Autodesk Inventor part; units mm, degrees
ref_plane "YZ Plane" through (0, 0, 0) normal (1, 0, 0) x (0, 1, 0)
ref_plane "XZ Plane" through (0, 0, 0) normal (0, 1, 0) x (-1, 0, 0)
ref_plane "XY Plane" through (0, 0, 0) normal (0, 0, 1) x (1, 0, 0)
sketch "Skizze1" plane through (0, 0, 0) normal (0, 1, 0) x (-1, 0, 0)
  line L0 (0, 0) -> (-110, 0)
  line L1 (-110, 0) -> (-110, 98)
  line L2 (-110, 98) -> (0, 98)
  line L3 (0, 98) -> (0, 0)
  dimension "d0" = 110
  dimension "d1" = 98
extrude "Extrusion1" add sketch "Skizze1" along normal blind 5
sketch "Skizze2" plane through (0, 0, 0) normal (0, -1, 0) x (1, 0, 0)
  line L0 (107, 93) -> (105, 93)
  line L1 (105, 93) -> (105, 36)
  line L2 (105, 36) -> (107, 36)
  line L3 (107, 36) -> (107, 93)
  line L4 (3, 93) -> (5, 93)
  line L5 (5, 93) -> (5, 36)
  line L6 (5, 36) -> (3, 36)
  line L7 (3, 36) -> (3, 93)
  line L8 (5, 36) -> (9, 36)
  line L9 (9, 36) -> (9, 38)
  line L10 (9, 38) -> (5, 38)
  line L11 (5, 38) -> (5, 36)
  line L12 (5, 93) -> (9, 93)
  line L13 (9, 93) -> (9, 91)
  line L14 (9, 91) -> (5, 91)
  line L15 (5, 91) -> (5, 93)
  line L16 (105, 93) -> (101, 93)
  line L17 (101, 93) -> (101, 91)
  line L18 (101, 91) -> (105, 91)
  line L19 (105, 91) -> (105, 93)
  line L20 (105, 36) -> (101, 36)
  line L21 (101, 36) -> (101, 38)
  line L22 (101, 38) -> (105, 38)
  line L23 (105, 38) -> (105, 36)
extrude "Extrusion2" add sketch "Skizze2" along normal blind 8 contours L3 L2 L1 L0
extrude "Extrusion3" add sketch "Skizze2" along normal blind 8 contours L20 L21 L22 L1
extrude "Extrusion4" add sketch "Skizze2" along normal blind 8 contours L1 L18 L17 L16
extrude "Extrusion5" add sketch "Skizze2" along normal blind 8 contours L5 L10 L9 L8
extrude "Extrusion6" add sketch "Skizze2" along normal blind 8 contours L4 L5 L6 L7
extrude "Extrusion7" add sketch "Skizze2" along normal blind 8 contours L12 L13 L14 L5
sketch "Skizze3" plane through (0, -8, 0) normal (0, -1, 0) x (1, 0, 0)
  line L0 (5, 38) -> (5, 91)
  line L1 (3, 93) -> (3, 36)
  line L2 (3, 80) -> (5, 80)
  line L3 (5, 80) -> (5, 50)
  line L4 (5, 50) -> (3, 50)
  line L5 (3, 50) -> (3, 80)
  point P0 (0, 0)
extrude "Extrusion8" cut sketch "Skizze3" against normal blind 8
sketch "Skizze4" plane through (0, 5, 0) normal (0, 1, 0) x (1, 0, 0)
  line L0 (12.0049, -91) -> (87.0387, -91)
  line L1 (87.0387, -91) -> (87.0387, -37.9492)
  line L2 (87.0387, -37.9492) -> (12.0049, -37.9492)
  line L3 (12.0049, -37.9492) -> (12.0049, -91)
extrude "Extrusion9" cut sketch "Skizze4" against normal blind 8
sketch "Skizze5" plane through (0, 0, 0) normal (0, -1, 0) x (1, 0, 0)
  line L0 (3, 3) -> (107, 3)
  line L1 (107, 3) -> (107, 30)
  line L2 (107, 30) -> (3, 30)
  line L3 (3, 30) -> (3, 3)
extrude "Extrusion10" add sketch "Skizze5" along normal blind 10
sketch "Skizze6" plane through (0, -10, 0) normal (0, -1, 0) x (1, 0, 0)
  line L0 (5, 5) -> (105, 5)
  line L1 (105, 5) -> (105, 28)
  line L2 (105, 28) -> (5, 28)
  line L3 (5, 28) -> (5, 5)
  point P0 (0, 0)
extrude "Extrusion11" cut sketch "Skizze6" against normal blind 10
sketch "Skizze7" plane through (0, -10, 0) normal (0, -1, 0) x (1, 0, 0)
  line L0 (107, 30) -> (3, 30)
  line L1 (5, 28) -> (105, 28)
  line L2 (14, 30) -> (98, 30)
  line L3 (98, 30) -> (98, 28)
  line L4 (98, 28) -> (14, 28)
  line L5 (14, 28) -> (14, 30)
  point P0 (0, 0)
extrude "Extrusion12" cut sketch "Skizze7" against normal blind 10
sketch "Skizze8" plane through (0, -10, 0) normal (0, -1, 0) x (1, 0, 0)
  line L0 (105, 5) -> (5, 5)
  line L1 (107, 3) -> (3, 3)
  line L2 (16, 5) -> (96, 5)
  line L3 (96, 5) -> (96, 3)
  line L4 (96, 3) -> (16, 3)
  line L5 (16, 3) -> (16, 5)
  point P0 (0, 0)
extrude "Extrusion13" cut sketch "Skizze8" against normal blind 10
sketch "Skizze14" plane through (0, 0, 0) normal (0, -1, 0) x (1, 0, 0)
  line L0 (87.0387, 37.9492) -> (98, 37.9492)
  line L1 (98, 37.9492) -> (98, 91)
  line L2 (98, 91) -> (87.0387, 91)
  line L3 (87.0387, 91) -> (87.0387, 37.9492)
extrude "Extrusion20" cut sketch "Skizze14" against normal blind 2
sketch "Skizze15" plane through (0, 0, 0) normal (0, -1, 0) x (1, 0, 0)
  line L0 (104, 6) -> (6, 6)
  line L1 (6, 6) -> (6, 27)
  line L2 (6, 27) -> (104, 27)
  line L3 (104, 27) -> (104, 6)
extrude "Extrusion21" cut sketch "Skizze15" against normal blind 3
sketch "Skizze16" plane through (0, -10, 0) normal (0, -1, 0) x (1, 0, 0)
  line L0 (104, 28) -> (6, 28)
  line L1 (6, 28) -> (6, 30)
  line L2 (6, 30) -> (104, 30)
  line L3 (104, 30) -> (104, 28)
  point P0 (0, 0)
extrude "Extrusion22" cut sketch "Skizze16" against normal blind 10
sketch "Skizze17" plane through (0, 0, 0) normal (0, -1, 0) x (1, 0, 0)
  line L0 (9, 36) -> (3, 36)
  line L1 (104, 27) -> (6, 27)
  line L2 (6, 27) -> (6, 36)
  line L3 (6, 36) -> (104, 36)
  line L4 (104, 36) -> (104, 27)
extrude "Extrusion23" cut sketch "Skizze17" against normal blind 3
sketch "Skizze18" plane through (0, 0, 0) normal (0, -1, 0) x (1, 0, 0)
  line L0 (12.0049, 91) -> (12.0049, 37.9492)
  line L1 (12.0049, 39) -> (6, 39)
  line L2 (6, 39) -> (6, 90)
  line L3 (6, 90) -> (12.0049, 90)
  line L4 (12.0049, 90) -> (12.0049, 39)
extrude "Extrusion24" cut sketch "Skizze18" against normal blind 3
properties part number "ARDUINO_DUE_CASE_TOP_NEU"
Build history of the part. All positions in model axes, mm. A direction names the side the tool comes from. Round coordinates to 2 decimals unless told otherwise and drop trailing zeros. Loops run counter-clockwise (first coordinate to the right, second up) from the corner with the lowest first, then second, coordinate; pieces in that order, holes last. Notation, with made-up numbers: M 32.5,-22.5 L 51.5,-22.5 A15 cw 51.5,5.5 Z; hole C 46.25,9.5 d4. An arc over 180 degrees is marked long. Answer as CSV lines item,"result".
1. Wall check: probe 1 along Z at (x, y) = (68, 0.5); probe 2 along X at (y, z) = (-5, 82.5); probe 3 along X at (y, z) = (1.5, 75). Give the ranges that are in metal, low to high. Write a range as [from, to].
Resolved:
probe 1,"z = [0, 6], [36, 37.95], [91, 98]"
probe 2,"x = [3, 5], [105, 107]"
probe 3,"x = [0, 6], [98, 110]"
2. Cut at A-A on z = 45.5. Write the cut outline in (x, y).
Resolved:
outline,"M 0,0 L 3,0 L 3,-8 L 5,-8 L 5,0 L 6,0 L 6,3 L 12,3 L 12,5 L 0,5 Z; M 87.04,2 L 98,2 L 98,0 L 105,0 L 105,-8 L 107,-8 L 107,0 L 110,0 L 110,5 L 87.04,5 Z"
3. Two-plate mould, pull along X, no slides. Class faces 4 (the flat face through (6, 1, 64)), 5 (the flat face through (106, -5, 30)), 6 (the flat face through (0, 2, 50)), 7 (the flat face through (54, 3, 91)): released by +X, released by -X, zero draft, split by the parting line, or undercut.
Resolved:
face 4,"undercut"
face 5,"zero draft"
face 6,"released by -X"
face 7,"undercut"
4. Cut at D-D on x = 92.5. Write the cut outline in (y, z).
Resolved:
outline,"M 0,0 L 5,0 L 5,98 L 0,98 L 0,91 L 2,91 L 2,37.95 L 0,37.95 L 0,36 L 3,36 L 3,6 L 0,6 Z"
5. Cut at C-C on z = 24.5. Write the cut outline in (x, y), then the cut area to 3 significant figures.
Resolved:
outline,"M 0,0 L 3,0 L 3,-10 L 5,-10 L 5,0 L 6,0 L 6,3 L 104,3 L 104,0 L 105,0 L 105,-10 L 107,-10 L 107,0 L 110,0 L 110,5 L 0,5 Z"
area,"296 mm²"
6. Cut at B-B on x = 79. Write the cut outline in (y, z).
Resolved:
outline,"M 0,0 L 5,0 L 5,37.95 L 0,37.95 L 0,36 L 3,36 L 3,6 L 0,6 Z; M 0,91 L 5,91 L 5,98 L 0,98 Z"
7. 3-axis set-ups, long thin cutter, end or side, ignore diameter. For faces 1 (the flat face through (9, 1, 39)), 2 (the flat face through (9, -5, 3)), 3 (the flat face through (87.039, 4, 65)): which of +Z, -Z, +X, -X, +Y, -Y reach the whole face in a straight line?
Resolved:
face 1,"-Y"
face 2,"-Z, +X, -X, -Y"
face 3,"+Y, -Y"
8. Flat gauge pins, fed straight in: P1, Ø1.1, axis at x = 5.5, y = -4.5, coming from the -Z side; P2, Ø8, axis at y = -8, z = 11.5, coming from the +X side; P3, Ø1.8, axis at x = 5.5, z = 40, coming from the -Y side. Where does each tip first touch, or does it go through?
Resolved:
P1,"stops at z = 3"
P2,"stops at x = 107"
P3,"stops at y = -8"
